For this review, take the finished solid that the model builds, in its own axes (mm). A direction names the side the tool comes from. Round coordinates to 2 decimals unless told otherwise and drop trailing zeros. Loops run counter-clockwise (first coordinate to the right, second up) from the corner with the lowest first, then second, coordinate; pieces in that order, holes last.
1) Take a section at A-A (y = -12). State the section outline as (x, z) points, then the cut area to 3 significant figures.
2) Take a section at D-D (z = 1.75). Give the number of separate pieces and of enclosed holes in the cut face, then the cut area to 3 significant figures.
3) Insertion check: pin 1 (8.5 mm diameter, centred on x = -87.25, y = 0, fed in from +Z); pin 2 (2.5 mm diameter, centred on x = -87.25, y = -12, fed in from +Z); pin 3 (1 mm diameter, centred on y = -5, z = 5, fed in from -X). Each pin has a flat end and moves straight along its axis. Give the tip position at first contact, or say it passes through.
4) Wall thickness on L1, parallel to X at y = -0.5, z = 7; L2, parallel to Y at x = 5.5, z = 2; L3, parallel to X at y = 8.5, z = 7.75: over which ranges is each line inside the solid? List them lowest first.
5) Take a section at C-C (y = 0). State the section outline as (x, z) points.
6) Tool access review of faces 1 (the cylindrical face through (-102.246, -0.33, 3.944)), 2 (the flat face through (-45, 10, 4)): name each direction out of +Z, -Z, +X, -X, +Y, -Y from which nothing blocks a thin tool from reaching the whole face with its end or side.
7) Mouldability with a two-part tool opening along X and no side actions: class faces 3 (the flat face through (-1, 15, 4)), 4 (the cylindrical face through (102.246, 0.33, 3.944)), 5 (the cylindrical face through (-78.209, -7.474, 3.944)) as pulls with the +X half, pulls with the -X half, needs draft (parallel to the pull), parting line crosses it, or undercut.
8) Take a section at B-B (x = 43). State the section outline as (y, z) points.
```python
from build123d import *

# Parameters (mm, degrees)
SKETCH1_R           = 6
BOSS_EXTRUDE1_DEPTH = 8
CIRPATTERN1_COUNT   = 6
SKETCH9_R           = 7
CUT_EXTRUDE1_DEPTH  = 4


with BuildPart() as part:
    # Sketch1 → Boss-Extrude1 (new body)
    with BuildSketch(Plane.XY):
        with BuildLine():
            Line((-87.25, 15), (87.25, 15))
            ThreePointArc((87.25, 15), (102.25, 0), (87.25, -15))
            Line((87.25, -15), (-87.25, -15))
            ThreePointArc((-87.25, -15), (-102.25, 0), (-87.25, 15))
        make_face()
        with Locations((87.25, 0)):
            Circle(SKETCH1_R, mode=Mode.SUBTRACT)
        with BuildLine():
            Line((61.25, -10), (38.75, -10))
            ThreePointArc((38.75, -10), (28.75, 0), (38.75, 10))
            Line((38.75, 10), (61.25, 10))
            ThreePointArc((61.25, 10), (71.25, 0), (61.25, -10))
        make_face(mode=Mode.SUBTRACT)
        with BuildLine():
            Line((13.75, -10), (-8.75, -10))
            ThreePointArc((-8.75, -10), (-18.75, 0), (-8.75, 10))
            Line((-8.75, 10), (13.75, 10))
            ThreePointArc((13.75, 10), (23.75, 0), (13.75, -10))
        make_face(mode=Mode.SUBTRACT)
        with BuildLine():
            Line((-33.75, -10), (-56.25, -10))
            ThreePointArc((-56.25, -10), (-66.25, 0), (-56.25, 10))
            Line((-56.25, 10), (-33.75, 10))
            ThreePointArc((-33.75, 10), (-23.75, 0), (-33.75, -10))
        make_face(mode=Mode.SUBTRACT)
    extrude(amount=BOSS_EXTRUDE1_DEPTH)

    # Sketch7 → 4.0mm Dowel Hole1 (revolve, cut)
    with BuildSketch(Plane(origin=(-87.25, 12, 0), x_dir=(0, 1, 0), z_dir=(1, 0, 0))):
        Polygon((0, 0), (0, 101.201721238), (2, 100), (2, 0), align=None)
    f_4_0mm_dowel_hole1 = revolve(axis=Axis((-87.25, 12, -6.35), (0, 0, 1)), mode=Mode.SUBTRACT)

    # CirPattern1: 4.0mm Dowel Hole1 ×6 about axis
    cirpattern1_axis = Axis((-87.25, 0, 0), (0, 0, 1))
    for i in range(1, CIRPATTERN1_COUNT):
        add(f_4_0mm_dowel_hole1.rotate(cirpattern1_axis, i * 360 / CIRPATTERN1_COUNT), mode=Mode.SUBTRACT)

    # Sketch9 → Cut-Extrude1 (cut)
    with BuildSketch(Plane.XY.offset(8)):
        with Locations((-87.25, 0)):
            Circle(SKETCH9_R)
    extrude(amount=-CUT_EXTRUDE1_DEPTH, mode=Mode.SUBTRACT)


solid = part.part
```
Response:
1. outline: (-96.25, 0) - (-89.25, 0) - (-89.25, 8) - (-96.25, 8) - close; (-85.25, 0) - (96.25, 0) - (96.25, 8) - (-85.25, 8) - close
1. area: 1,510 mm2
2. separate pieces: 1
2. enclosed holes: 10
2. area: 3,460 mm2
3. pin 1: stops at z = 4
3. pin 2: passes through
3. pin 3: stops at x = -101.56
4. L1: x = -102.24 to -94.23, -80.27 to -66.24, -23.76 to -18.74, 23.74 to 28.76, 71.24 to 81.27, 93.23 to 102.24
4. L2: y = -15 to -10, 10 to 15
4. L3: x = -99.61 to -61.52, -28.48 to -14.02, 19.02 to 33.48, 66.52 to 99.61
5. outline: (-102.25, 0) - (-66.25, 0) - (-66.25, 8) - (-80.25, 8) - (-80.25, 4) - (-94.25, 4) - (-94.25, 8) - (-102.25, 8) - close; (-23.75, 0) - (-18.75, 0) - (-18.75, 8) - (-23.75, 8) - close; (23.75, 0) - (28.75, 0) - (28.75, 8) - (23.75, 8) - close; (71.25, 0) - (81.25, 0) - (81.25, 8) - (71.25, 8) - close; (93.25, 0) - (102.25, 0) - (102.25, 8) - (93.25, 8) - close
6. face 1: +Z, -Z, -X
6. face 2: +Z, -Z
7. face 3: needs draft
7. face 4: pulls with the +X half
7. face 5: undercut
8. outline: (-15, 0) - (-10, 0) - (-10, 8) - (-15, 8) - close; (10, 0) - (15, 0) - (15, 8) - (10, 8) - close
